For this review, take the finished solid that the model builds, in its own axes (mm). A direction names the side the tool comes from. Coordinates: 2 decimals unless noted, no trailing zeros. Loops run counter-clockwise (first coordinate to the right, second up) from the corner with the lowest first, then second, coordinate; pieces in that order, holes last. Notation, with made-up numbers: (78.5, 89.5) - (97.5, 89.5) arc R16 cw to (97.5, 94.5) - close; hole circle Ø5 at (-38.75, -7). An arc over 180 degrees is marked (long way). Use one line per item in the form item = value. Start each with the question number.
1. Machinability: for faces 4 (the face through (-22.72, -2.75, -12.4)), 5 (the face through (70.59, -0.69, -3.1)), 6 (the face through (-12.7, 5, 0)), which of the approach directions +Z, -Z, +X, -X, +Y, -Y give a long, thin tool a straight path to every point of the face, cutting with its end or side? Answer none if there is none.
2. For pin 1 Ø1 at (y, z) = (3, 3) entering from +X; pin 2 Ø7.5 at (y, z) = (6, 0) entering from +X; pin 3 Ø1 at (x, y) = (84.5, -3) entering from +Z; pin 4 Ø4 at (x, y) = (-13, -8.5) entering from -Z, all flat-tipped, find the tip position at first contact; note any pin that passes through.
3. To check wall thickness, follow probe 1 along X at (y, z) = (-7.75, 6.75); probe 2 along Y at (x, z) = (-16.5, -0.75); probe 3 along Y at (x, z) = (33.5, -1.25). State the ranges of each line that lie inside material, in increasing order.
4. Add section A-A on z = 10.75. Give the boundary of the cut face in (x, y), and give its area (3 significant figures).
5. Add section C-C on y = 0. Give the boundary of the cut face in (x, z) (1 decimal), and give its area (3 significant figures).
6. Add section D-D on x = 92. Give the boundary of the cut face in (y, z) (3 decimals).
7. Add section B-B on y = 7.5. Give the boundary of the cut face in (x, z), and give its area (3 significant figures).
8. Draft analysis for pull direction X (two halves, no side actions). For faces 1 (the face through (109.22, 0, 0)), 2 (the face through (22.72, -2.75, -12.4)), 3 (the face through (12.7, 5, 0)), state which applies: +X half, -X half, draft (parallel to the pull), parting line (faces both ways), or undercut.
```python
from build123d import *

# Parameters (mm, degrees)
F0_R     = 4.7625
F1_DEPTH = 12.7
F2_R     = 12.7
F3_DEPTH = 20.32
F5_R     = 3.175
F6_DEPTH = 76.2


with BuildPart() as f1:
    # F0 (on Right) → F1 (new body)
    with BuildSketch(Plane.YZ):
        Circle(F0_R)
    extrude(amount=F1_DEPTH)

    # F2 (on face) → F3 (join)
    with BuildSketch(Plane.YZ.offset(12.7)):
        Circle(F2_R)
    extrude(amount=F3_DEPTH)

    # F4: F1 across plane


with BuildPart() as f1_1:
    add(f1.part)
    add(f1.part.mirror(Plane.YZ))

    # F5 (on face) → F6 (join)
    with BuildSketch(Plane.YZ.offset(33.02)):
        Circle(F5_R)
    extrude(amount=F6_DEPTH)


solid = f1_1.part
```
Conclusion:
q1.face_4 = +X, -X
q1.face_5 = +X
q1.face_6 = none
q2.pin_1 = 33.02
q2.pin_2 = 109.22
q2.pin_3 = 1.96
q2.pin_4 = -10.91
q3.probe_1 = -33.02 to -12.7, 12.7 to 33.02
q3.probe_2 = -12.68 to 12.68
q3.probe_3 = -2.92 to 2.92
q4.outline = (-33.02, -6.76) - (-12.7, -6.76) - (-12.7, 6.76) - (-33.02, 6.76) - close; (12.7, -6.76) - (33.02, -6.76) - (33.02, 6.76) - (12.7, 6.76) - close
q4.area = 550 mm^2
q5.outline = (-33, -12.7) - (-12.7, -12.7) - (-12.7, -4.8) - (12.7, -4.8) - (12.7, -12.7) - (33, -12.7) - (33, -3.2) - (109.2, -3.2) - (109.2, 3.2) - (33, 3.2) - (33, 12.7) - (12.7, 12.7) - (12.7, 4.8) - (-12.7, 4.8) - (-12.7, 12.7) - (-33, 12.7) - close
q5.area = 1,760 mm^2
q6.outline = circle Ø6.35 at (0, 0)
q7.outline = (-33.02, -10.25) - (-12.7, -10.25) - (-12.7, 10.25) - (-33.02, 10.25) - close; (12.7, -10.25) - (33.02, -10.25) - (33.02, 10.25) - (12.7, 10.25) - close
q7.area = 833 mm^2
q8.face_1 = +X half
q8.face_2 = draft
q8.face_3 = undercut
